Autodesk Inventor part; units mm, degrees
ref_plane "YZ Plane" through (0, 0, 0) normal (1, 0, 0) x (0, 1, 0)
ref_plane "XZ Plane" through (0, 0, 0) normal (0, 1, 0) x (-1, 0, 0)
ref_plane "XY Plane" through (0, 0, 0) normal (0, 0, 1) x (1, 0, 0)
sketch "Sketch1" plane through (0, 0, 0) normal (0, 1, 0) x (-1, 0, 0)
  circle A0 centre (0, 0) radius 3
  dimension "d0" = 6
extrude "Extrusion1" add sketch "Sketch1" along normal blind 39.8
hole "Hole1" at (0, 0, 0) direction (0, 1, 0) diameter 4.2 depth 6
sketch "Sketch2" plane through (0, 39.8, 0) normal (0, 1, 0) x (1, 0, 0)
  point P0 (0, 0)
hole "Hole2" at (0, 39.8, 0) direction (0, -1, 0) diameter 4.2 depth 6
properties part number "Dribbler Support"
Geometry: final body of the model. Coordinates: model frame, mm. A direction names the side the tool comes from. Coordinates: 2 decimals unless noted, no trailing zeros. Write each loop counter-clockwise with the first axis right and the second up, starting at its lowest first coordinate (ties: lowest second). Pieces come first, ordered by that corner, then holes. Notation, with made-up numbers: (-9.75, 34.5) - (4.25, 34.5) arc R21 ccw to (4.25, 64.5) - close; hole circle Ø1 at (44, 64). An arc over 180 degrees is marked (long way). Return JSON: item names as keys, results as strings.
Item 1: Reachability of faces 1 (the face through (0, 33.8, 0)), 2 (the face through (-0.631, 3.042, -2.003)), 3 (the face through (-1.3, 39.8, -2)) from +Z, -Z, +X, -X, +Y, -Y: full face, straight path, thin tool, end or side. Return the list, or none.
Completed:
{"face 1": "+Y", "face 2": "-Y", "face 3": "+Z, -Z, +X, -X, +Y"}
Item 2: Section query B-B (x = 0). Output: boundary loops of the cut face in (y, z).
Completed:
{"outline": "(0, -3) - (39.8, -3) - (39.8, -2.1) - (33.8, -2.1) - (33.8, 2.1) - (39.8, 2.1) - (39.8, 3) - (0, 3) - (0, 2.1) - (6, 2.1) - (6, -2.1) - (0, -2.1) - close"}
Item 3: Pull-direction query (X, two-part tool) for faces 4 (the face through (0, 6, 0)), 5 (the face through (-1.3, 0, -2)), 6 (the face through (3, 20, 0)); classes: +X half, -X half, draft (parallel to the pull), parting line (faces both ways), or undercut.
Completed:
{"face 4": "undercut", "face 5": "draft", "face 6": "parting line"}
Item 4: Section query D-D (y = 18). Output: boundary loops of the cut face in (x, z), and give its area (3 significant figures).
Completed:
{"outline": "circle Ø6 at (0, 0)", "area": "28.3 mm2"}
Item 5: Section query A-A (z = 0). Output: boundary loops of the cut face in (x, y), and give its area (3 significant figures).
Completed:
{"outline": "(-3, 0) - (-2.1, 0) - (-2.1, 6) - (2.1, 6) - (2.1, 0) - (3, 0) - (3, 39.8) - (2.1, 39.8) - (2.1, 33.8) - (-2.1, 33.8) - (-2.1, 39.8) - (-3, 39.8) - close", "area": "188 mm2"}
Item 6: Line query: L1, parallel to Z at x = 0, y = 36.2; L2, parallel to Y at x = -1.6, z = -1.05; L3, parallel to X at y = 34, z = -1.55. Output: solid intervals per line, ascending.
Completed:
{"L1": "z = -3 to -2.1, 2.1 to 3", "L2": "y = 6 to 33.8", "L3": "x = -2.57 to -1.42, 1.42 to 2.57"}
Item 7: Section query C-C (y = 34.5). Output: boundary loops of the cut face in (x, z).
Completed:
{"outline": "circle Ø6 at (0, 0); hole circle Ø4.2 at (0, 0)"}
Item 8: Pin query (flat end, axial travel): pin 1 Ø3.5 at (x, z) = (0, 0) entering from -Y. Return the tip coordinate at first contact, or that it passes through.
Completed:
{"pin 1": "stops at y = 6"}
